Drawing for the job (mm, zero at the part's lowest x, y, z). Coordinates: 2 decimals unless noted, no trailing zeros. Order: outer loops, then holes, each group sorted by start corner. A loop starts at its lowest first (then second) coordinate and runs counter-clockwise, first axis right, second up. Notation, with made-up numbers: M -13.75,76.25 L 44.25,76.25 A28 cw 44.25,114.25 Z; hole C -28,84 d5. An arc over 180 degrees is marked long. Write item = value, one per line. Start each with the question number.
Q1. Drill centre lines: probe 1 along Y at (x, z) = (43, 12); probe 2 along Z at (x, y) = (9.5, 68.5); probe 3 along Y at (x, z) = (51.5, 44). Where is each one in solid material? Low to high.
Q2. Band-saw the part on A-A on y = 43. Write the cut outline in (x, z), plus the area to 3 significant figures.
Q3. Pull direction Z, two halves, no side cores. Call the marked faces 1, 2 and 3: released by +Z, released by -Z, zero draft, split by the parting line, or undercut.
Q4. Band-saw the part on C-C on z = 52.5. Write the cut outline in (x, y).
Q5. Pin check, flat tips, straight feed: P1, Ø1.5, axis at x = 73.5, z = 33.5, coming from the -Y side; P2, Ø3, axis at x = 43, y = 58, coming from the +Z side; P3, Ø10, axis at y = 44.5, z = 40.5, coming from the +X side; P4, Ø5, axis at y = 26.5, z = 38, coming from the -X side. Stop position of each tip, or through.
Q6. Band-saw the part on D-D on x = 58. Write the cut outline in (y, z), plus the area to 3 significant figures.
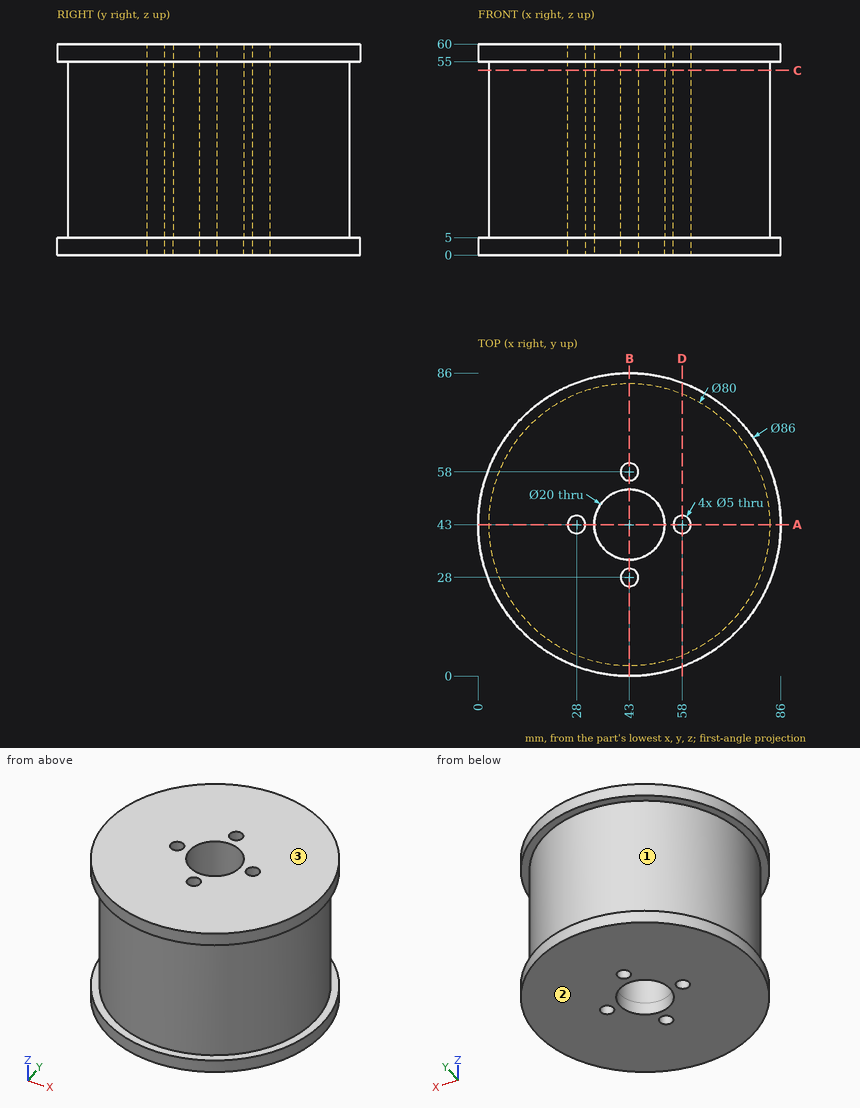
Recorded:
q1.probe_1 = 3 to 25.5, 30.5 to 33, 53 to 55.5, 60.5 to 83
q1.probe_2 = 0 to 5, 55 to 60
q1.probe_3 = 3.91 to 37.73, 48.27 to 82.09
q2.outline = M 0,0 L 25.5,0 L 25.5,60 L 0,60 L 0,55 L 3,55 L 3,5 L 0,5 Z; M 30.5,0 L 33,0 L 33,60 L 30.5,60 Z; M 53,0 L 55.5,0 L 55.5,60 L 53,60 Z; M 60.5,0 L 86,0 L 86,5 L 83,5 L 83,55 L 86,55 L 86,60 L 60.5,60 Z
q2.area = 3,060 mm2
q3.face_1 = undercut
q3.face_2 = released by -Z
q3.face_3 = released by +Z
q4.outline = C 43,43 d80; hole C 28,43 d5; hole C 43,43 d20; hole C 43,28 d5; hole C 43,58 d5; hole C 58,43 d5
q5.P1 = 16.26
q5.P2 = through
q5.P3 = 83
q5.P4 = 5.53
q6.outline = M 2.7,0 L 40.5,0 L 40.5,60 L 2.7,60 L 2.7,55 L 5.92,55 L 5.92,5 L 2.7,5 Z; M 45.5,0 L 83.3,0 L 83.3,5 L 80.08,5 L 80.08,55 L 83.3,55 L 83.3,60 L 45.5,60 Z
q6.area = 4,210 mm2
